```python
from build123d import *

# Parameters (mm, degrees)
EXTRUDE_2_DEPTH      = 10
SKETCH_5_R           = 1.6
CUT_EXTRUDE_1_DEPTH  = 27
SKETCH_8_R           = 8
EXTRUDE_4_DEPTH      = 10
SKETCH_8_3_R         = 8
CUT_EXTRUDE_4_DEPTH  = 4.62
SKETCH_10_R          = 5
CUT_EXTRUDE_6_DEPTH  = 33.62
CUT_EXTRUDE_7_DEPTH  = 33.62
EXTRUDE_5_DEPTH      = 3
SKETCH_13_R          = 8
CUT_EXTRUDE_8_DEPTH  = 1.4
CUT_EXTRUDE_10_DEPTH = 6.02


with BuildPart() as part:
    # 草图4 → 凸台-拉伸2 (new body)
    with BuildSketch(Plane.XY):
        with BuildLine():
            Line((-9.472780877, 3.204125849), (-7.330319061, 3.204125849))
            ThreePointArc((-7.330319061, 3.204125849), (0, 8), (7.330319061, 3.204125849))
            Line((7.330319061, 3.204125849), (9.472780877, 3.204125849))
            ThreePointArc((9.472780877, 3.204125849), (0, 10), (-9.472780877, 3.204125849))
        make_face()
        with BuildLine():
            Line((9.472780877, 3.204125849), (7.330319061, 3.204125849))
            ThreePointArc((7.330319061, 3.204125849), (7.83079027, 1.636680712), (8, 0))
            ThreePointArc((8, 0), (7.83079027, -1.636680712), (7.330319061, -3.204125849))
            Line((7.330319061, -3.204125849), (9.472780877, -3.204125849))
            Line((9.472780877, -3.204125849), (9.472780877, 3.204125849))
        make_face()
        with BuildLine():
            ThreePointArc((7.330319061, -3.204125849), (0, -8), (-7.330319061, -3.204125849))
            Line((-7.330319061, -3.204125849), (-9.472780877, -3.204125849))
            ThreePointArc((-9.472780877, -3.204125849), (0, -10), (9.472780877, -3.204125849))
            Line((9.472780877, -3.204125849), (7.330319061, -3.204125849))
        make_face()
        with BuildLine():
            ThreePointArc((-7.330319061, -3.204125849), (-8, 0), (-7.330319061, 3.204125849))
            Line((-7.330319061, 3.204125849), (-9.472780877, 3.204125849))
            Line((-9.472780877, 3.204125849), (-9.472780877, -3.204125849))
            Line((-9.472780877, -3.204125849), (-7.330319061, -3.204125849))
        make_face()
    extrude(amount=EXTRUDE_2_DEPTH)

    # 草图5 → 切除-拉伸1 (cut)
    with BuildSketch(Plane.ZY.offset(9.472780877)):
        with Locations((3, 0)):
            Circle(SKETCH_5_R)
    extrude(amount=-CUT_EXTRUDE_1_DEPTH, mode=Mode.SUBTRACT)

    # 草图8 → 凸台-拉伸4 (add)
    with BuildSketch(Plane(origin=(0, 0, 0), x_dir=(-1, 0, 0), z_dir=(0, 0, -1))):
        Circle(SKETCH_8_R)
    extrude(amount=-EXTRUDE_4_DEPTH)

    # 草图8<3> → 切除-拉伸4 (cut)
    with BuildSketch(Plane(origin=(0, 0, 0), x_dir=(-1, 0, 0), z_dir=(0, 0, -1))):
        Circle(SKETCH_8_3_R)
    extrude(amount=-CUT_EXTRUDE_4_DEPTH, mode=Mode.SUBTRACT)

    # 草图10 → 切除-拉伸6 (cut)
    with BuildSketch(Plane.XY.offset(10)):
        Circle(SKETCH_10_R)
    extrude(amount=-CUT_EXTRUDE_6_DEPTH, mode=Mode.SUBTRACT)

    # 草图11 → 切除-拉伸7 (cut)
    with BuildSketch(Plane.XY.offset(10)):
        with BuildLine():
            ThreePointArc((5, 0), (4.639856446, -1.863258479), (3.611307136, -3.458100746))
            Line((3.611307136, -3.458100746), (5, -3.458100746))
            Line((5, -3.458100746), (5, 0))
        make_face()
        with BuildLine():
            Line((5, 3.204125849), (3.838434257, 3.204125849))
            ThreePointArc((3.838434257, 3.204125849), (4.700647364, 1.704087544), (5, 0))
            Line((5, 0), (5, 3.204125849))
        make_face()
        with BuildLine():
            Line((-3.838434257, 3.204125849), (-5, 3.204125849))
            Line((-5, 3.204125849), (-5, 0))
            ThreePointArc((-5, 0), (-4.700647364, 1.704087544), (-3.838434257, 3.204125849))
        make_face()
        with BuildLine():
            ThreePointArc((-3.611307136, -3.458100746), (-4.639856446, -1.863258479), (-5, 0))
            Line((-5, 0), (-5, -3.458100746))
            Line((-5, -3.458100746), (-3.611307136, -3.458100746))
        make_face()
    extrude(amount=-CUT_EXTRUDE_7_DEPTH, mode=Mode.SUBTRACT)

    # 草图14 → 凸台-拉伸5 (add)
    with BuildSketch(Plane.XY.offset(10)):
        with BuildLine():
            Line((-9.472780877, 3.204125849), (-9.472780877, -3.204125849))
            ThreePointArc((-9.472780877, -3.204125849), (0, -10), (9.472780877, -3.204125849))
            Line((9.472780877, -3.204125849), (9.472780877, 3.204125849))
            ThreePointArc((9.472780877, 3.204125849), (0, 10), (-9.472780877, 3.204125849))
        make_face()
        with BuildLine():
            ThreePointArc((-3.838434257, 3.204125849), (0, 5), (3.838434257, 3.204125849))
            Line((3.838434257, 3.204125849), (5, 3.204125849))
            Line((5, 3.204125849), (5, -3.458100746))
            Line((5, -3.458100746), (3.611307136, -3.458100746))
            ThreePointArc((3.611307136, -3.458100746), (0, -5), (-3.611307136, -3.458100746))
            Line((-3.611307136, -3.458100746), (-5, -3.458100746))
            Line((-5, -3.458100746), (-5, 3.204125849))
            Line((-5, 3.204125849), (-3.838434257, 3.204125849))
        make_face(mode=Mode.SUBTRACT)
    extrude(amount=EXTRUDE_5_DEPTH)

    # 草图13 → 切除-拉伸8 (cut)
    with BuildSketch(Plane(origin=(0, 0, 4.62), x_dir=(-1, 0, 0), z_dir=(0, 0, -1))):
        Circle(SKETCH_13_R)
        with BuildLine():
            Line((-5, -3.458100746), (-3.611307136, -3.458100746))
            ThreePointArc((-3.611307136, -3.458100746), (0, -5), (3.611307136, -3.458100746))
            Line((3.611307136, -3.458100746), (5, -3.458100746))
            Line((5, -3.458100746), (5, 3.204125849))
            Line((5, 3.204125849), (3.838434257, 3.204125849))
            ThreePointArc((3.838434257, 3.204125849), (0, 5), (-3.838434257, 3.204125849))
            Line((-3.838434257, 3.204125849), (-5, 3.204125849))
            Line((-5, 3.204125849), (-5, -3.458100746))
        make_face(mode=Mode.SUBTRACT)
    extrude(amount=-CUT_EXTRUDE_8_DEPTH, mode=Mode.SUBTRACT)

    # 草图15 → 切除-拉伸10 (cut)
    with BuildSketch(Plane(origin=(0, 0, 0), x_dir=(-1, 0, 0), z_dir=(0, 0, -1))):
        Polygon((-8, 3.204125849), (-8, -3.204125849), (8, -3.204125849), (8, 3.204125849), (-7.888349605, 3.204125849), align=None)
    extrude(amount=-CUT_EXTRUDE_10_DEPTH, mode=Mode.SUBTRACT)


solid = part.part
```
For this review, take the finished solid that the model builds, in its own axes (mm). A direction names the side the tool comes from. Coordinates: 2 decimals unless noted, no trailing zeros. Write each loop counter-clockwise with the first axis right and the second up, starting at its lowest first coordinate (ties: lowest second). Pieces come first, ordered by that corner, then holes. Notation, with made-up numbers: (-16.75, 12.5) -> (37.25, 12.5) arc R23 cw to (37.25, 28.5) -> close; hole circle Ø8 at (68, 69). An arc over 180 degrees is marked (long way). Put each result on its own line as item: value.
Q1. Take a section at B-B, the plane z = 3. State the section outline as (x, y) points, then the cut area to 3 significant figures.
From the geometry:
outline: (-9.47, -3.2) arc R10 ccw to (9.47, -3.2) -> (9.47, -1.6) -> (8, -1.6) -> (8, -3.2) -> (7.33, -3.2) arc R8 cw to (-7.33, -3.2) -> (-8, -3.2) -> (-8, -1.6) -> (-9.47, -1.6) -> close; (-9.47, 1.6) -> (-8, 1.6) -> (-8, 3.2) -> (-7.33, 3.2) arc R8 cw to (7.33, 3.2) -> (8, 3.2) -> (8, 1.6) -> (9.47, 1.6) -> (9.47, 3.2) arc R10 ccw to (-9.47, 3.2) -> close
area: 96.3 mm2
Q2. Wall thickness on L1, parallel to X at y = -0.25, z = 0.5; L2, parallel to Z at x = -8.55, y = 0; L3, parallel to X at y = 3, z = 10: over which ranges is each line inside the solid? List them lowest first.
From the geometry:
L1: x = -9.47 to -8, 8 to 9.47
L2: z = 0 to 1.4, 4.6 to 13
L3: x = -9.47 to -5, 5 to 9.47
Q3. Tool access review of faces 4 (the flat face through (-4, 3.204, 9)), 5 (the cylindrical face through (0, 10, 6)), 6 (the cylindrical face through (0, -8, 3)): name each direction out of +Z, -Z, +X, -X, +Y, -Y from which nothing blocks a thin tool from reaching the whole face with its end or side.
From the geometry:
face 4: +Z, -Z
face 5: +Z, -Z, +Y
face 6: -Z
Q4. Clearance check with flat-ended pins moving along their axes: pin 1 Ø6 at (x, z) = (-6.5, 7) entering from -Y; pin 2 Ø1.1 at (x, z) = (4, 7) entering from +Y; pin 3 Ø3 at (y, z) = (0, 3) entering from +X; pin 4 Ø6 at (y, z) = (7, 8) entering from -X. State where each tip first meets the part, or that it passes through.
From the geometry:
pin 1: stops at y = -9.37
pin 2: stops at y = 9.39
pin 3: passes through
pin 4: stops at x = -9.17
Q5. The part is to be moulded in two halves that separate along Z. For faces 1 (the flat face through (-9.473, 0, 6)), 2 (the cylindrical face through (8.73, 0.07, 1.4)), 3 (the flat face through (-5.2, 0.1, 6.02)), say which applies: +Z half, -Z half, draft (parallel to the pull), parting line (faces both ways), or undercut.
From the geometry:
face 1: draft
face 2: undercut
face 3: -Z half
Q6. Take a section at A-A, the plane y = 0. State the section outline as (x, z) points, then the cut area to 3 significant figures.
From the geometry:
outline: (-9.47, 0) -> (-8, 0) -> (-8, 1.4) -> (-9.47, 1.4) -> close; (-9.47, 4.6) -> (-8, 4.6) -> (-8, 6.02) -> (-5, 6.02) -> (-5, 13) -> (-9.47, 13) -> close; (5, 6.02) -> (8, 6.02) -> (8, 4.6) -> (9.47, 4.6) -> (9.47, 13) -> (5, 13) -> close; (8, 0) -> (9.47, 0) -> (9.47, 1.4) -> (8, 1.4) -> close
area: 70.7 mm2
Q7. Take a section at D-D, the plane x = -4.5. State the section outline as (y, z) points.
From the geometry:
outline: (-8.93, 0) -> (-6.61, 0) -> (-6.61, 6.02) -> (-3.46, 6.02) -> (-3.46, 13) -> (-8.93, 13) -> close; (3.2, 6.02) -> (6.61, 6.02) -> (6.61, 0) -> (8.93, 0) -> (8.93, 13) -> (3.2, 13) -> close
Q8. Take a section at C-C, the plane z = 12.25. State the section outline as (x, y) points.
From the geometry:
outline: (-9.47, -3.2) arc R10 ccw to (9.47, -3.2) -> (9.47, 3.2) arc R10 ccw to (-9.47, 3.2) -> close; hole (-5, -3.46) -> (-3.61, -3.46) arc R5 ccw to (3.61, -3.46) -> (5, -3.46) -> (5, 3.2) -> (3.84, 3.2) arc R5 ccw to (-3.84, 3.2) -> (-5, 3.2) -> close
